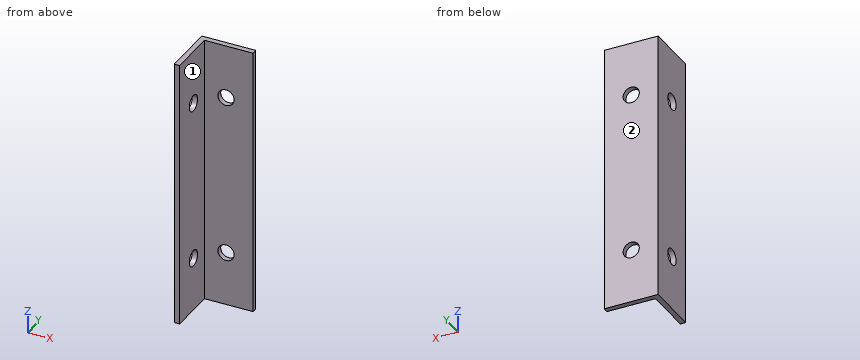
from build123d import *

# Parameters (mm, degrees)
BOSS_EXTRUDE1_DEPTH = 100
SKETCH3_R           = 3
CUT_EXTRUDE1_DEPTH  = 20
SKETCH4_R           = 3
CUT_EXTRUDE2_DEPTH  = 20
SKETCH5_R           = 3
CUT_EXTRUDE3_DEPTH  = 20
SKETCH6_R           = 3
CUT_EXTRUDE4_DEPTH  = 20


with BuildPart() as part:
    # Sketch2 → Boss-Extrude1 (new body)
    with BuildSketch(Plane.XY):
        Polygon((0, 0), (0, 20), (20, 20), (20, 18), (2, 18), (2, 0), align=None)
    extrude(amount=BOSS_EXTRUDE1_DEPTH)

    # Sketch3 → Cut-Extrude1 (cut)
    with BuildSketch(Plane.ZY):
        with Locations((80, 10)):
            Circle(SKETCH3_R)
    extrude(amount=-CUT_EXTRUDE1_DEPTH, mode=Mode.SUBTRACT)

    # Sketch4 → Cut-Extrude2 (cut)
    with BuildSketch(Plane.ZY):
        with Locations((20, 10)):
            Circle(SKETCH4_R)
    extrude(amount=-CUT_EXTRUDE2_DEPTH, mode=Mode.SUBTRACT)

    # Sketch5 → Cut-Extrude3 (cut)
    with BuildSketch(Plane(origin=(0, 20, 0), x_dir=(1, 0, 0), z_dir=(0, 1, 0))):
        with Locations((10, -80)):
            Circle(SKETCH5_R)
    extrude(amount=-CUT_EXTRUDE3_DEPTH, mode=Mode.SUBTRACT)

    # Sketch6 → Cut-Extrude4 (cut)
    with BuildSketch(Plane(origin=(0, 20, 0), x_dir=(1, 0, 0), z_dir=(0, 1, 0))):
        with Locations((10, -20)):
            Circle(SKETCH6_R)
    extrude(amount=-CUT_EXTRUDE4_DEPTH, mode=Mode.SUBTRACT)


solid = part.part
Model file for the job. Use its own axes, mm. Face numbers are marked on the shaded views. A direction names the side the tool comes from. Give positions to 0.01 mm unless a question says otherwise; leave off trailing zeros. Write each loop counter-clockwise with the first axis right and the second up, starting at its lowest first coordinate (ties: lowest second). Pieces come first, ordered by that corner, then holes. Notation, with made-up numbers: M 63,58 L 72,58 A17 ccw 72,65 Z; hole C 76.5,-20.75 d3. An arc over 180 degrees is marked long. One line per item, written item: value. Start each with the question number.
Q1. Drop flat-ended pins along their axis: pin 1 Ø5.5 at (x, z) = (13.5, 67.5) entering from -Y; pin 2 Ø12 at (y, z) = (4.5, 71) entering from +X. Give the stop position or say it passes through.
Q2. Saw through at A-A, the plane y = 10. Write the cut outline in (x, z).
Q3. Saw through at B-B, the plane x = 10. Write the cut outline in (y, z).
Q4. Saw through at C-C, the plane z = 20. Write the cut outline in (x, y), plus the area to 3 significant figures.
Q5. 3-axis set-ups, long thin cutter, end or side, ignore diameter. For the marked faces 1 and 2: which of +Z, -Z, +X, -X, +Y, -Y reach the whole face in a straight line?
Q6. Saw through at D-D, the plane z = 63. Write the cut outline in (x, y), plus the area to 3 significant figures.
Q7. Probe probe 1 along Z at (x, y) = (10, 19.5); probe 2 along X at (y, z) = (19.5, 80). List the from-to ranges inside material, lowest first. Write a range as [from, to].
Output values:
1. pin 1: stops at y = 18
1. pin 2: stops at x = 2
2. outline: M 0,0 L 2,0 L 2,17 L 0,17 Z; M 0,23 L 2,23 L 2,77 L 0,77 Z; M 0,83 L 2,83 L 2,100 L 0,100 Z
3. outline: M 18,0 L 20,0 L 20,17 L 18,17 Z; M 18,23 L 20,23 L 20,77 L 18,77 Z; M 18,83 L 20,83 L 20,100 L 18,100 Z
4. outline: M 0,0 L 2,0 L 2,7 L 0,7 Z; M 0,13 L 2,13 L 2,18 L 7,18 L 7,20 L 0,20 Z; M 13,18 L 20,18 L 20,20 L 13,20 Z
4. area: 52.0 mm²
5. face 1: +Z, -Z, +X, -Y
5. face 2: +Z, -Z, +X, -X, +Y
6. outline: M 0,0 L 2,0 L 2,18 L 20,18 L 20,20 L 0,20 Z
6. area: 76.0 mm²
7. probe 1: z = [0, 17], [23, 77], [83, 100]
7. probe 2: x = [0, 7], [13, 20]
